```python
from build123d import *

# Parameters (mm, degrees)
SKETCH001_R       = 0.05
EXTRUDE001_DEPTH  = 2
BOX017_W          = 21
BOX017_H          = 13.5
BOX017_DEPTH      = 5
FILLET006_R       = 1
BOX007_W          = 21
BOX007_H          = 13.5
BOX007_DEPTH      = 10
FILLET004_R       = 1
BOX006_W          = 16.5
BOX006_H          = 10
BOX006_DEPTH      = 13.25
BOX005_W          = 31
BOX005_H          = 27
BOX005_DEPTH      = 25
CYLINDER004_R     = 6.5
CYLINDER004_DEPTH = 10
BOX014_W          = 27
BOX014_H          = 20
BOX014_DEPTH      = 27.5
BOX013_W          = 78.5
BOX013_H          = 108.5
BOX013_DEPTH      = 37
FILLET003_R       = 3
BOX018_W          = 20.8
BOX018_H          = 13.3
BOX018_DEPTH      = 5
FILLET007_R       = 1
BOX016_W          = 20.8
BOX016_H          = 13.3
BOX016_DEPTH      = 10
FILLET005_R       = 1


with BuildPart() as extrude001:
    # Sketch001 → Extrude001 (new body)
    with BuildSketch(Plane(origin=(0, 0, 0), x_dir=(1, 0, 0), z_dir=(0, 0, -1))):
        with BuildLine():
            ThreePointArc((10.5, -19.625), (8.625, -21.5), (10.5, -23.375))
            Line((10.5, -23.375), (13.04, -23.375))
            ThreePointArc((13.04, -23.375), (15.998193, -25.004413), (18.956385, -23.375))
            Line((18.956385, -23.375), (21.5, -23.375))
            ThreePointArc((21.5, -23.375), (23.375, -21.5), (21.5, -19.625))
            Line((21.5, -19.625), (18.955398, -19.625))
            ThreePointArc((18.955398, -19.625), (16, -18), (13.044602, -19.625))
            Line((13.044602, -19.625), (10.5, -19.625))
        make_face()
        with Locations((16, -21.5)):
            Circle(SKETCH001_R, mode=Mode.SUBTRACT)
        with BuildLine():
            ThreePointArc((55.25, -75.625), (53.375, -77.5), (55.25, -79.375))
            Line((55.25, -79.375), (57.794602, -79.375))
            ThreePointArc((57.794602, -79.375), (60.752301, -81.003632), (63.71, -79.375))
            Line((63.71, -79.375), (66.25, -79.375))
            ThreePointArc((66.25, -79.375), (68.125, -77.5), (66.25, -75.625))
            Line((66.25, -75.625), (63.705398, -75.625))
            ThreePointArc((63.705398, -75.625), (60.75, -74), (57.794602, -75.625))
            Line((57.794602, -75.625), (55.25, -75.625))
        make_face()
        with Locations((60.75, -77.5)):
            Circle(SKETCH001_R, mode=Mode.SUBTRACT)
    extrude(amount=EXTRUDE001_DEPTH)


with BuildPart() as extrude001_1:
    # Extrude001 placement: moved
    add(extrude001.part.moved(Location((0, 0, 2))))


with BuildPart() as key_hole001:
    # Box017 → Box017 (new body)
    with BuildSketch(Plane(origin=(5.5, 13.5, 0), x_dir=(1, 0, 0), z_dir=(0, 0, 1))):
        with Locations((10.5, 6.75)):
            Rectangle(BOX017_W, BOX017_H)
    extrude(amount=BOX017_DEPTH)

    # Fillet006
    fillet006_edges = [key_hole001.edges().sort_by_distance(p)[0] for p in [
        (5.5, 13.5, 2.5),
        (5.5, 27, 2.5),
        (26.5, 13.5, 2.5),
        (26.5, 27, 2.5),
    ]]
    fillet(fillet006_edges, radius=FILLET006_R)


with BuildPart() as key_hole001_1:
    # Fillet006 placement: moved
    add(key_hole001.part.moved(Location((45, 57.75, 0))))


with BuildPart() as key_hole:
    # Box007 → Box007 (new body)
    with BuildSketch(Plane(origin=(5.5, 15, 0), x_dir=(1, 0, 0), z_dir=(0, 0, 1))):
        with Locations((10.5, 6.75)):
            Rectangle(BOX007_W, BOX007_H)
    extrude(amount=BOX007_DEPTH)

    # Fillet004
    fillet004_edges = [key_hole.edges().sort_by_distance(p)[0] for p in [
        (5.5, 15, 5),
        (5.5, 28.5, 5),
        (26.5, 15, 5),
        (26.5, 28.5, 5),
    ]]
    fillet(fillet004_edges, radius=FILLET004_R)


with BuildPart() as obj1:
    # Box006 → Box006 (new body)
    with BuildSketch(Plane(origin=(11.25, 101, 14.8), x_dir=(1, 0, 0), z_dir=(0, 0, 1))):
        with Locations((8.25, 5)):
            Rectangle(BOX006_W, BOX006_H)
    extrude(amount=BOX006_DEPTH)


with BuildPart() as cube009:
    # Box005 → Box005 (new body)
    with BuildSketch(Plane(origin=(37.5, 83.5, 6), x_dir=(1, 0, 0), z_dir=(0, 0, 1))):
        with Locations((15.5, 13.5)):
            Rectangle(BOX005_W, BOX005_H)
    extrude(amount=BOX005_DEPTH)


with BuildPart() as cylinder004:
    # Cylinder004 → Cylinder004 (new body)
    with BuildSketch(Plane(origin=(61, 31, 27), x_dir=(1, 0, 0), z_dir=(0, 0, 1))):
        Circle(CYLINDER004_R)
    extrude(amount=CYLINDER004_DEPTH)


with BuildPart() as cube001:
    # Box014 → Box014 (new body)
    with BuildSketch(Plane(origin=(26.5, 0, 4.75), x_dir=(1, 0, 0), z_dir=(0, 0, 1))):
        with Locations((13.5, 10)):
            Rectangle(BOX014_W, BOX014_H)
    extrude(amount=BOX014_DEPTH)


with BuildPart() as hole2:
    # Box013 → Box013 (new body)
    with BuildSketch(Plane.XY):
        with Locations((39.25, 54.25)):
            Rectangle(BOX013_W, BOX013_H)
    extrude(amount=BOX013_DEPTH)

    # Cut001: cut Cube001
    add(cube001.part, mode=Mode.SUBTRACT)

    # Cut002: cut Cylinder004
    add(cylinder004.part, mode=Mode.SUBTRACT)

    # Cut006: cut Cube009
    add(cube009.part, mode=Mode.SUBTRACT)

    # Cut007: cut obj1
    add(obj1.part, mode=Mode.SUBTRACT)

    # Fillet003
    fillet003_edges = [hole2.edges().sort_by_distance(p)[0] for p in [
        (0, 0, 18.5),
        (0, 54.25, 37),
        (0, 108.5, 18.5),
        (0, 54.25, 0),
        (39.25, 0, 0),
        (78.5, 0, 18.5),
        (39.25, 0, 37),
        (39.25, 108.5, 37),
        (78.5, 54.25, 37),
        (39.25, 108.5, 0),
        (78.5, 108.5, 18.5),
        (78.5, 54.25, 0),
    ]]
    fillet(fillet003_edges, radius=FILLET003_R)

    # Cut008: cut Key_hole
    add(key_hole.part, mode=Mode.SUBTRACT)

    # Cut009: cut Key_hole001
    add(key_hole001_1.part, mode=Mode.SUBTRACT)


with BuildPart() as key_hole002:
    # Box018 → Box018 (new body)
    with BuildSketch(Plane(origin=(5.5, 13.5, 0), x_dir=(1, 0, 0), z_dir=(0, 0, 1))):
        with Locations((10.4, 6.65)):
            Rectangle(BOX018_W, BOX018_H)
    extrude(amount=BOX018_DEPTH)

    # Fillet007
    fillet007_edges = [key_hole002.edges().sort_by_distance(p)[0] for p in [
        (5.5, 13.5, 2.5),
        (5.5, 26.8, 2.5),
        (26.3, 13.5, 2.5),
        (26.3, 26.8, 2.5),
    ]]
    fillet(fillet007_edges, radius=FILLET007_R)


with BuildPart() as key_hole002_1:
    # Fillet007 placement: moved
    add(key_hole002.part.moved(Location((45.1, 57.85, 0))))


with BuildPart() as cut010:
    # Box016 → Box016 (new body)
    with BuildSketch(Plane(origin=(5.6, 15.1, 0), x_dir=(1, 0, 0), z_dir=(0, 0, 1))):
        with Locations((10.4, 6.65)):
            Rectangle(BOX016_W, BOX016_H)
    extrude(amount=BOX016_DEPTH)

    # Fillet005
    fillet005_edges = [cut010.edges().sort_by_distance(p)[0] for p in [
        (5.6, 15.1, 5),
        (5.6, 28.4, 5),
        (26.4, 15.1, 5),
        (26.4, 28.4, 5),
    ]]
    fillet(fillet005_edges, radius=FILLET005_R)

    # Fusion007: union Hole2, Key_hole002
    add(hole2.part)
    add(key_hole002_1.part)

    # Cut010: cut Extrude001
    add(extrude001_1.part, mode=Mode.SUBTRACT)


solid = cut010.part
```
Part model, mm, in its own coordinate system. Round coordinates to 2 decimals unless told otherwise and drop trailing zeros. Loops run counter-clockwise (first coordinate to the right, second up) from the corner with the lowest first, then second, coordinate; pieces in that order, holes last.
Item 1: Cut at B-B, the plane z = 22. Give the cut face in (x, y).
Item 2: Cut at D-D, the plane x = 34.5. Give the cut face in (y, z), then the cut area to 3 significant figures.
Item 3: Mould opens along Z. For faces 1 (the face through (0.86, 54.97, 36.1)), 2 (the face through (78.5, 54, 18)), 3 (the face through (53, 96, 6)), 4 (the face through (14, 25, 0)) say: +Z half, -Z half, draft (parallel to the pull), parting line (faces both ways), or undercut.
Item 4: Drop flat-ended pins along their axis: P1, Ø2, axis at x = 19.5, z = 1, coming from the +Y side; P2, Ø2, axis at x = 16, y = 20.5, coming from the -Z side; P3, Ø6, axis at x = 55, z = 14.5, coming from the +Y side; P4, Ø1, axis at x = 20, z = 1, coming from the -Y side. Give the stop position or say it passes through.
Item 5: Cut at C-C, the plane y = 31. Give the cut face in (x, z), then the cut area to 3 significant figures.
Item 6: Drill centre lines: line 1 (X direction, y = 103.5, z = 22.5); line 2 (X direction, y = 9, z = 31.5); line 3 (Y direction, x = 61, z = 32.5). Where is each one in solid material? Low to high.
Item 7: Cut at A-A, the plane y = 87. Give the cut face in (x, z), then the cut area to 3 significant figures.
A:
1. outline: (0, 3) arc R3 ccw to (3, 0) - (26.5, 0) - (26.5, 20) - (53.5, 20) - (53.5, 0) - (75.5, 0) arc R3 ccw to (78.5, 3) - (78.5, 105.5) arc R3 ccw to (75.5, 108.5) - (68.5, 108.5) - (68.5, 83.5) - (37.5, 83.5) - (37.5, 108.5) - (27.75, 108.5) - (27.75, 101) - (11.25, 101) - (11.25, 108.5) - (3, 108.5) arc R3 ccw to (0, 105.5) - close
2. outline: (0, 3) arc R3 ccw to (3, 0) - (105.5, 0) arc R3 ccw to (108.5, 3) - (108.5, 34) arc R3 ccw to (105.5, 37) - (3, 37) arc R3 ccw to (0, 34) - (0, 32.25) - (20, 32.25) - (20, 4.75) - (0, 4.75) - close
2. area: 3,460 mm2
3. face 1: +Z half
3. face 2: draft
3. face 3: undercut
3. face 4: -Z half
4. P1: stops at y = 108.33
4. P2: stops at z = 0
4. P3: stops at y = 83.5
4. P4: stops at y = 0.4
5. outline: (0, 3) arc R3 ccw to (3, 0) - (75.5, 0) arc R3 ccw to (78.5, 3) - (78.5, 34) arc R3 ccw to (75.5, 37) - (67.5, 37) - (67.5, 27) - (54.5, 27) - (54.5, 37) - (3, 37) arc R3 ccw to (0, 34) - close
5. area: 2,770 mm2
6. line 1: x = 0 to 11.25, 27.75 to 37.5, 68.5 to 78.5
6. line 2: x = 0 to 26.5, 53.5 to 78.5
6. line 3: y = 0 to 24.5, 37.5 to 108.5
7. outline: (0, 3) arc R3 ccw to (3, 0) - (75.5, 0) arc R3 ccw to (78.5, 3) - (78.5, 34) arc R3 ccw to (75.5, 37) - (3, 37) arc R3 ccw to (0, 34) - close; hole (37.5, 6) - (68.5, 6) - (68.5, 31) - (37.5, 31) - close
7. area: 2,120 mm2
